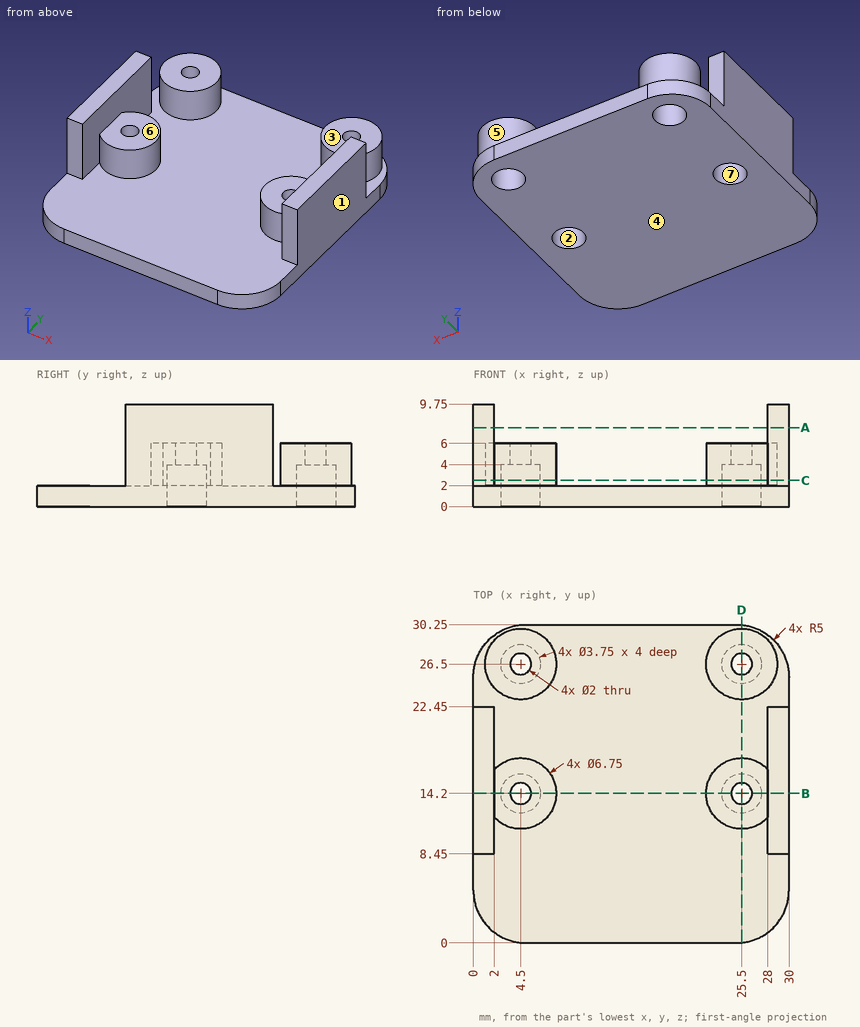
Geometry check sheet. Reference: drawing and pictorial views, mm from the part's lowest x, y, z. A direction names the side the tool comes from. Round coordinates to 2 decimals unless told otherwise and drop trailing zeros. Order: outer loops, then holes, each group sorted by start corner. A loop starts at its lowest first (then second) coordinate and runs counter-clockwise, first axis right, second up. Notation, with made-up numbers: M 14,76.25 L 66,76.25 A21 ccw 66,90.25 Z; hole C 85.25,-16 d10. An arc over 180 degrees is marked long. Write item = value, one per line.
Q1. Section check D-D (x = 25.5). Enter the section's corners in (y, z) (3 decimals), plus the area to 3 significant figures.
Answer block:
outline = M 0.025,0 L 12.325,0 L 12.325,4 L 13.2,4 L 13.2,6 L 10.825,6 L 10.825,2 L 0.025,2 Z; M 15.2,4 L 16.075,4 L 16.075,0 L 24.625,0 L 24.625,4 L 25.5,4 L 25.5,6 L 23.125,6 L 23.125,2 L 17.575,2 L 17.575,6 L 15.2,6 Z; M 27.5,4 L 28.375,4 L 28.375,0 L 30.225,0 L 30.225,2 L 29.875,2 L 29.875,6 L 27.5,6 Z
area = 76.4 mm^2
Q2. Depth check by flat-ended pin: pin 1 Ø3 at (y, z) = (27, 8) entering from -X; pin 2 Ø2.5 at (x, y) = (4.5, 14.2) entering from -Z; pin 3 Ø3 at (x, y) = (4.5, 26.5) entering from +Z; pin 4 Ø10 at (x, y) = (15.5, 12.5) entering from +Z. Enter the tip coordinate at first touch or a pass-through.
Answer block:
pin_1 = through
pin_2 = 4
pin_3 = 6
pin_4 = 2
Q3. Section check A-A (z = 7.5). Enter the section's corners in (x, y), plus the area to 3 significant figures.
Answer block:
outline = M 0,8.45 L 2,8.45 L 2,22.45 L 0,22.45 Z; M 28,8.45 L 30,8.45 L 30,22.45 L 28,22.45 Z
area = 56.0 mm^2
Q4. Section check C-C (z = 2.5). Enter the section's corners in (x, y) (3 decimals), plus the area to 3 significant figures.
Answer block:
outline = M 0,8.45 L 2,8.45 L 2,11.933 A3.375 ccw long 2,16.467 L 2,22.45 L 0,22.45 Z; C 4.5,26.5 d6.75; C 25.5,26.5 d6.75; M 28,8.45 L 30,8.45 L 30,22.45 L 28,22.45 L 28,16.467 A3.375 ccw long 28,11.933 Z; hole C 4.5,14.2 d3.75; hole C 4.5,26.5 d3.75; hole C 25.5,14.2 d3.75; hole C 25.5,26.5 d3.75
area = 150 mm^2
Q5. Scan lines: line 1 (Y direction, x = 25.5, z = 5.05) (3 decimals); line 2 (X direction, y = 14.2, z = 5.1) (3 decimals); line 3 (X direction, y = 26.5, z = 5.1) (3 decimals). Record each from-to range of solid material in increasing order.
Answer block:
line_1 = 10.825 to 13.2, 15.2 to 17.575, 23.125 to 25.5, 27.5 to 29.875
line_2 = 0 to 3.5, 5.5 to 7.875, 22.125 to 24.5, 26.5 to 30
line_3 = 1.125 to 3.5, 5.5 to 7.875, 22.125 to 24.5, 26.5 to 28.875
Q6. Section check B-B (y = 14.2). Enter the section's corners in (x, z) (3 decimals), plus the area to 3 significant figures.
Answer block:
outline = M 0,0 L 2.625,0 L 2.625,4 L 3.5,4 L 3.5,6 L 2,6 L 2,9.75 L 0,9.75 Z; M 5.5,4 L 6.375,4 L 6.375,0 L 23.625,0 L 23.625,4 L 24.5,4 L 24.5,6 L 22.125,6 L 22.125,2 L 7.875,2 L 7.875,6 L 5.5,6 Z; M 26.5,4 L 27.375,4 L 27.375,0 L 30,0 L 30,9.75 L 28,9.75 L 28,6 L 26.5,6 Z
area = 100 mm^2
Q7. Set-up check for the marked faces 4, 5, 6 and 7: record each of +Z, -Z, +X, -X, +Y, -Y from which the full face is reachable in a straight line by a thin tool's end or side.
Answer block:
face_4 = -Z, +X, -X, +Y, -Y
face_5 = +Z
face_6 = +Z, +Y, -Y
face_7 = -Z
Q8. Release check for a two-part mould opening along X. For the marked faces 1, 2 and 3 record: released by +X, released by -X, zero draft, split by the parting line, or undercut.
Answer block:
face_1 = released by +X
face_2 = undercut
face_3 = zero draft
